The listing builds one solid part. Answer for the finished solid, in the listing's coordinates (mm). A direction names the side the tool comes from. Round coordinates to 2 decimals unless told otherwise and drop trailing zeros. Order: outer loops, then holes, each group sorted by start corner. A loop starts at its lowest first (then second) coordinate and runs counter-clockwise, first axis right, second up. Notation, with made-up numbers: (28, 26.5) -> (73, 26.5) arc R20 cw to (73, 46.5) -> close; hole circle Ø11 at (-24, -34.75). An arc over 180 degrees is marked (long way). Answer in a Markdown table with one row per item. Add a question column.
```python
from build123d import *

# Parameters (mm, degrees)
EXTRUDE_THIN1_DEPTH = 46.863
BOSS_EXTRUDE1_START = 3.175
BOSS_EXTRUDE1_DEPTH = 3.175
FILLET1_START       = -50.038
FILLET1_DEPTH       = 100.076
FILLET2_START       = -50.038
FILLET2_DEPTH       = 100.076
SKETCH4_W           = 30.9245
SKETCH4_H           = 20.6375
CUT_EXTRUDE1_DEPTH  = 3.175


with BuildPart() as part:
    # Sketch2 → Extrude-Thin1 (new, symmetric)
    with BuildSketch(Plane(origin=(0, 0, 0), x_dir=(0, 0, -1), z_dir=(1, 0, 0))):
        with BuildLine():
            Line((0, 0), (0, 14.2875))
            ThreePointArc((0, 14.2875), (0.92993597, 16.53256403), (3.175, 17.4625))
            Line((3.175, 17.4625), (49.149, 17.4625))
            ThreePointArc((49.149, 17.4625), (51.39406403, 16.53256403), (52.324, 14.2875))
            Line((52.324, 14.2875), (52.324, 0))
            Line((52.324, 0), (50.292, 0))
            Line((50.292, 0), (50.292, 14.2875))
            ThreePointArc((50.292, 14.2875), (49.957223051, 15.095723051), (49.149, 15.4305))
            Line((49.149, 15.4305), (3.175, 15.4305))
            ThreePointArc((3.175, 15.4305), (2.366776949, 15.095723051), (2.032, 14.2875))
            Line((2.032, 14.2875), (2.032, 0))
            Line((2.032, 0), (0, 0))
        make_face()
    extrude(amount=EXTRUDE_THIN1_DEPTH, both=True)

    # Sketch3 → Boss-Extrude1 (add)
    with BuildSketch(Plane(origin=(46.863, 0, 0), x_dir=(0, 0, -1), z_dir=(1, 0, 0)).offset(BOSS_EXTRUDE1_START)):
        with BuildLine():
            Line((52.324, 20.6375), (3.175, 20.6375))
            ThreePointArc((3.175, 20.6375), (-1.315128061, 18.777628061), (-3.175, 14.2875))
            Line((-3.175, 14.2875), (-3.175, 0))
            Line((-3.175, 0), (0, 0))
            Line((0, 0), (2.032, 0))
            Line((2.032, 0), (2.032, 14.2875))
            ThreePointArc((2.032, 14.2875), (2.366776949, 15.095723051), (3.175, 15.4305))
            Line((3.175, 15.4305), (49.149, 15.4305))
            ThreePointArc((49.149, 15.4305), (49.957223051, 15.095723051), (50.292, 14.2875))
            Line((50.292, 14.2875), (50.292, 0))
            Line((50.292, 0), (52.324, 0))
            Line((52.324, 0), (52.324, 14.2875))
            Line((52.324, 14.2875), (52.324, 20.6375))
        make_face()
    boss_extrude1 = extrude(amount=-BOSS_EXTRUDE1_DEPTH)

    # Mirror1: Boss-Extrude1 across plane
    add(boss_extrude1.mirror(Plane(origin=(0, 0, 0), x_dir=(0, 0, 1), z_dir=(1, 0, 0))))

    # Fillet1: read off the stored shape, not the designer's step
    # Fillet1 outline → Fillet1 (add)
    with BuildSketch(Plane.YZ.offset(FILLET1_START)):
        with BuildLine():
            ThreePointArc((15.4305, -47.117), (14.50056403, -49.36206403), (12.2555, -50.292))
            Line((12.2555, -50.292), (14.2875, -50.292))
            ThreePointArc((14.2875, -50.292), (15.095723051, -49.957223051), (15.4305, -49.149))
            Line((15.4305, -49.149), (15.4305, -47.117))
        make_face()
    extrude(amount=FILLET1_DEPTH)

    # Fillet2: read off the stored shape, not the designer's step
    # Fillet2 outline → Fillet2 (add)
    with BuildSketch(Plane.YZ.offset(FILLET2_START)):
        with BuildLine():
            ThreePointArc((12.2555, -2.032), (14.50056403, -2.96193597), (15.4305, -5.207))
            Line((15.4305, -5.207), (15.4305, -3.175))
            ThreePointArc((15.4305, -3.175), (15.095723051, -2.366776949), (14.2875, -2.032))
            Line((14.2875, -2.032), (12.2555, -2.032))
        make_face()
    extrude(amount=FILLET2_DEPTH)

    # Sketch4 → Cut-Extrude1 (cut)
    with BuildSketch(Plane(origin=(50.038, 0, 0), x_dir=(0, 0, -1), z_dir=(1, 0, 0))):
        with Locations((12.28725, 10.31875)):
            Rectangle(SKETCH4_W, SKETCH4_H)
    extrude(amount=-CUT_EXTRUDE1_DEPTH, mode=Mode.SUBTRACT)


solid = part.part
```
1. For faces 1 (the flat face through (46.863, 16, -9)), 2 (the flat face through (-1, 6, -50.292)), 3 (the cylindrical face through (0.656, 16.557, -51.369)), 4 (the flat face through (-1, 6, -52.324)), 5 (the flat face through (-48, 7, 3.175)), determine the directions among +Z, -Z, +X, -X, +Y, -Y from which every point of the face is accessible in a straight line to the end or side of a thin tool.
2. The part is cut by section C-C (z = -37). Give the vertices of the cut face in (x, y), then the cut area to 3 significant figures.
3. The mould has two halves that part along X. Classify faces 6 (the flat face through (50.038, 16, -43)), 7 (the cylindrical face through (0.7, 16.5, -0.9)), 8 (the flat face through (-50.038, 16, -24)), 9 (the flat face through (1, 17.462, -26)): released by +X, released by -X, zero draft, split by the parting line, or undercut.
4. Straight lines are drawn through the part: line 1 along Z through (x, y) = (-44, 4.25); line 2 along Y through (x, z) = (-45, -32.5); line 3 along X through (y, z) = (19, -18). For each, find the intervals that lie inside material, in ascending order.
5. The part is cut by section D-D (z = -16). Give the vertices of the cut face in (x, y).
6. The part is cut by section A-A (y = 8.25). Give the vertices of the cut face in (x, z) (3 decimals).
7. Each of these flat-tipped pins is pushed along its axis until it touches: pin 1 (3 mm diameter, centred on x = 28, y = 11.5, fed in from +Z); pin 2 (1 mm diameter, centred on x = -4, z = -14.5, fed in from -Y); pin 3 (2.5 mm diameter, centred on x = 49, y = 18, fed in from +Z). Where does it stop, or does it pass through?
Report:
| question | item | result |
|---|---|---|
| 1 | face 1 | +Z, +X, +Y, -Y |
| 1 | face 2 | +X, -X, -Y |
| 1 | face 3 | -Z, +Y |
| 1 | face 4 | -Z, +X, -X, +Y, -Y |
| 1 | face 5 | +Z, +X, -X, +Y, -Y |
| 2 | outline | (-50.04, 15.43) -> (50.04, 15.43) -> (50.04, 20.64) -> (46.86, 20.64) -> (46.86, 17.46) -> (-46.86, 17.46) -> (-46.86, 20.64) -> (-50.04, 20.64) -> close |
| 2 | area | 224 mm^2 |
| 3 | face 6 | released by +X |
| 3 | face 7 | zero draft |
| 3 | face 8 | released by -X |
| 3 | face 9 | undercut |
| 4 | line 1 | z = -52.32 to -50.29, -2.03 to 0 |
| 4 | line 2 | y = 15.43 to 17.46 |
| 4 | line 3 | x = -50.04 to -46.86 |
| 5 | outline | (-50.04, 15.43) -> (46.86, 15.43) -> (46.86, 17.46) -> (-46.86, 17.46) -> (-46.86, 20.64) -> (-50.04, 20.64) -> close |
| 6 | outline | (-50.038, -52.324) -> (50.038, -52.324) -> (50.038, -50.292) -> (-50.038, -50.292) -> close; (-50.038, -2.032) -> (46.863, -2.032) -> (46.863, 0) -> (-46.863, 0) -> (-46.863, 3.175) -> (-50.038, 3.175) -> close |
| 7 | pin 1 | stops at z = 0 |
| 7 | pin 2 | stops at y = 15.43 |
| 7 | pin 3 | stops at z = -27.75 |
